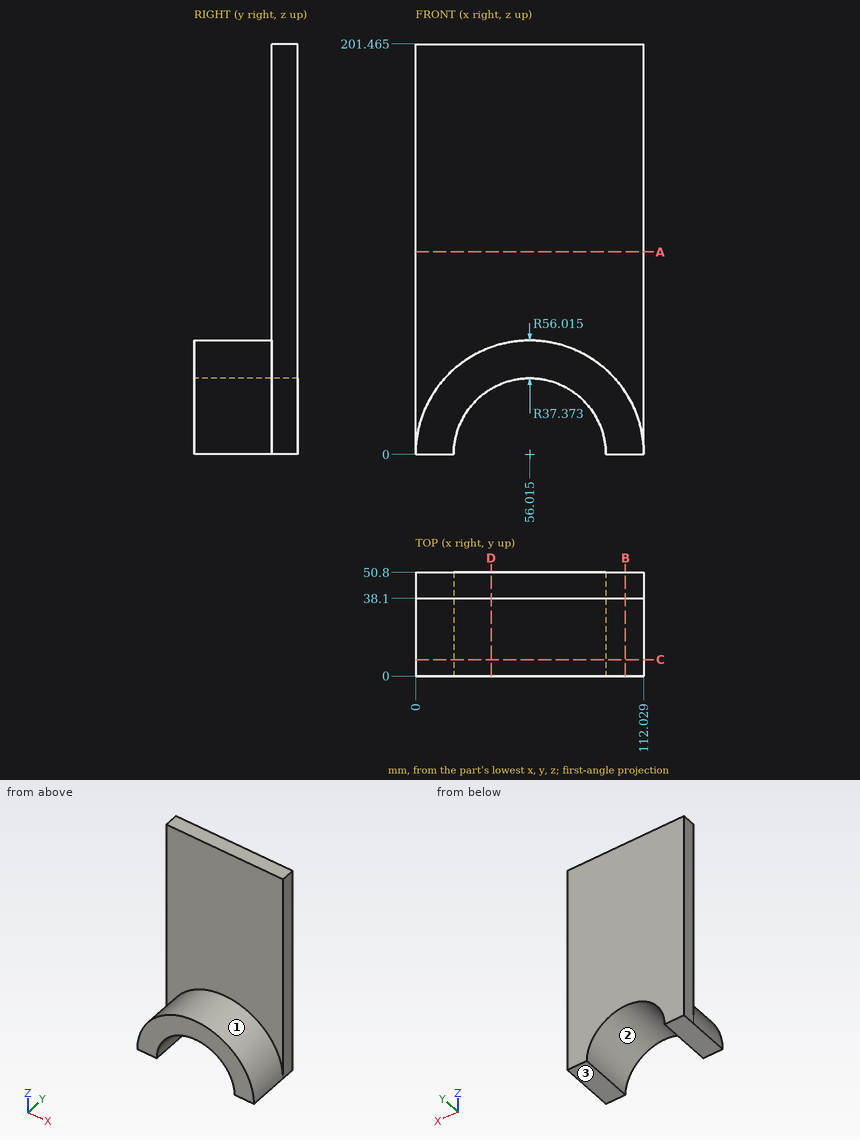
Study the drawing (mm; zero at the part's minimum x, y, z) and answer. Give positions to 0.01 mm unless a question says otherwise; leave off trailing zeros. Order: outer loops, then holes, each group sorted by start corner. A loop starts at its lowest first (then second) coordinate and runs counter-clockwise, first axis right, second up.
1. Each of these flat-tipped pins is pushed along its axis until it touches: P1, Ø1, axis at y = 38, z = 166.5, coming from the +X side; P2, Ø4, axis at x = 36, z = 179.5, coming from the -Y side; P3, Ø8, axis at y = 9, z = 46.5, coming from the -X side (1 decimal). Where does it stop, or does it pass through?
Result sheet:
P1: stops at x = 112.03
P2: stops at y = 38.1
P3: stops at x = 19.5
2. The mould has two halves that part along X. Classify the marked faces 1, 2 and 3: released by +X, released by -X, zero draft, split by the parting line, or undercut.
Result sheet:
face 1: split by the parting line
face 2: undercut
face 3: zero draft
3. Section A-A, the plane z = 99.5 is taken. Determine the outline of the cut face in (x, y), and give its area (3 significant figures).
Result sheet:
outline: (0, 38.1) - (112.03, 38.1) - (112.03, 50.8) - (0, 50.8) - close
area: 1,420 mm2
4. Straight lines are drawn through the part: L1, parallel to Y at x = 68.5, z = 170.5; L2, parallel to X at y = 19, z = 10 (1 decimal); L3, parallel to Z at x = 79.5, y = 5 (1 decimal). For each, find the intervals that lie inside material, in ascending order.
Result sheet:
L1: y = 38.1 to 50.8
L2: x = 0.9 to 20, 92 to 111.1
L3: z = 29.1 to 50.9
5. Section D-D, the plane x = 37 is taken. Determine the outline of the cut face in (y, z) (1 decimal).
Result sheet:
outline: (0, 32.2) - (50.8, 32.2) - (50.8, 201.5) - (38.1, 201.5) - (38.1, 52.7) - (0, 52.7) - close
6. Section C-C, the plane y = 8 is taken. Determine the outline of the cut face in (x, z) (1 decimal).
Result sheet:
outline: (0, 0) - (18.6, 0) arc R37.4 cw to (93.4, 0) - (112, 0) arc R56 ccw to start
7. Section B-B, the plane x = 103 is taken. Determine the outline of the cut face in (y, z) (1 decimal), and give its area (3 significant figures).
Result sheet:
outline: (0, 0) - (50.8, 0) - (50.8, 201.5) - (38.1, 201.5) - (38.1, 30.5) - (0, 30.5) - close
area: 3,720 mm2
